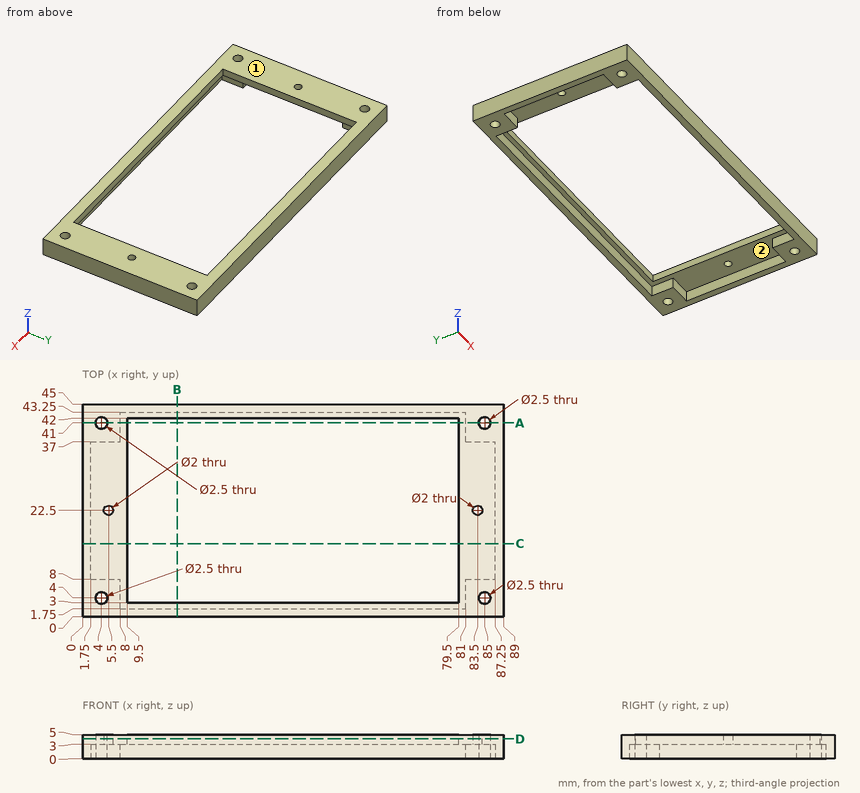
Verification items for this drawing (mm, ordinates from the low corner). Coordinates: 2 decimals unless noted, no trailing zeros. Loops run counter-clockwise (first coordinate to the right, second up) from the corner with the lowest first, then second, coordinate; pieces in that order, holes last. Notation, with made-up numbers: (79.25, 59) - (133.25, 59) arc R25 ccw to (133.25, 87) - close; hole circle Ø8 at (15, 37.25). An arc over 180 degrees is marked (long way). Use one line per item in the form item = value. Start each with the question number.
Item 1: Section check B-B, the plane x = 20. Enter the section's corners in (y, z).
Item 2: Section check D-D, the plane z = 4.15. Enter the section's corners in (x, y).
Item 3: Gauge pin test, flat end, axial feed: pin 1 (2.5 mm diameter, centred on x = 83.5, y = 22.5, fed in from -Z). Record the tip position at first contact, or that the pin passes through.
Item 4: Section check A-A, the plane y = 41. Enter the section's corners in (x, z), and give its area (3 significant figures).
Item 5: Thickness scan on probe 1 along Y at (x, z) = (4, 3.9); probe 2 along Y at (x, z) = (4, 2.25); probe 3 along X at (y, z) = (41, 1.45). Record the ranges inside material, lowest first.
Item 6: Mould release check, pull along X, two halves, no side actions. Record for the marked faces 1 and 2: +X half, -X half, draft (parallel to the pull), parting line (faces both ways), or undercut.
Item 7: Section check C-C, the plane y = 15.5. Enter the section's corners in (x, z), and give its area (3 significant figures).
Computed:
q1.outline = (0, 0) - (1.75, 0) - (1.75, 3) - (3, 3) - (3, 5) - (0, 5) - close; (42, 3) - (43.25, 3) - (43.25, 0) - (45, 0) - (45, 5) - (42, 5) - close
q2.outline = (0, 0) - (89, 0) - (89, 45) - (0, 45) - close; hole circle Ø2.5 at (4, 4); hole circle Ø2.5 at (4, 41); hole circle Ø2 at (5.5, 22.5); hole (9.5, 3) - (79.5, 3) - (79.5, 42) - (9.5, 42) - close; hole circle Ø2 at (83.5, 22.5); hole circle Ø2.5 at (85, 4); hole circle Ø2.5 at (85, 41)
q3.pin_1 = 3
q4.outline = (0, 0) - (2.75, 0) - (2.75, 5) - (0, 5) - close; (5.25, 0) - (8, 0) - (8, 3) - (9.5, 3) - (9.5, 5) - (5.25, 5) - close; (79.5, 3) - (81, 3) - (81, 0) - (83.75, 0) - (83.75, 5) - (79.5, 5) - close; (86.25, 0) - (89, 0) - (89, 5) - (86.25, 5) - close
q4.area = 61.0 mm2
q5.probe_1 = 0 to 2.75, 5.25 to 39.75, 42.25 to 45
q5.probe_2 = 0 to 2.75, 5.25 to 8, 37 to 39.75, 42.25 to 45
q5.probe_3 = 0 to 2.75, 5.25 to 8, 81 to 83.75, 86.25 to 89
q6.face_1 = draft
q6.face_2 = undercut
q7.outline = (0, 0) - (1.75, 0) - (1.75, 3) - (9.5, 3) - (9.5, 5) - (0, 5) - close; (79.5, 3) - (87.25, 3) - (87.25, 0) - (89, 0) - (89, 5) - (79.5, 5) - close
q7.area = 48.5 mm2
